```python
from build123d import *

# Parameters (mm, degrees)
BOSS_EXTRUDE1_DEPTH                              = 20.32
BOSS_EXTRUDE2_DEPTH                              = 12.7
CBORE_FOR_10_PAN_HEAD_MACHINE_SCREW1_D           = 5.08
CBORE_FOR_10_PAN_HEAD_MACHINE_SCREW1_CBORE_D     = 12.7
CBORE_FOR_10_PAN_HEAD_MACHINE_SCREW1_CBORE_DEPTH = 3.3782
FILLET1_R                                        = 5.08
FILLET2_R                                        = 2.54
FILLET3_R                                        = 2.54
FILLET4_R                                        = 2.54


with BuildPart() as part:
    # Sketch1 → Boss-Extrude1 (new, symmetric)
    with BuildSketch(Plane(origin=(0, 0, 0), x_dir=(0, 0, -1), z_dir=(1, 0, 0))):
        Polygon((0, 0), (0, 127), (-10.16, 127), (-10.16, 19.05), (-76.2, 19.05), (-76.2, 31.75), (-88.9, 31.75), (-88.9, 0), align=None)
    extrude(amount=BOSS_EXTRUDE1_DEPTH, both=True)

    # Sketch1<9> → Boss-Extrude2 (add, symmetric)
    with BuildSketch(Plane(origin=(0, 0, 0), x_dir=(0, 0, -1), z_dir=(1, 0, 0))):
        Polygon((-54.61, 19.05), (-10.16, 80.01), (-10.16, 67.31), (-45.349583333, 19.05), align=None)
    extrude(amount=BOSS_EXTRUDE2_DEPTH, both=True)

    # CBORE for #10 Pan Head Machine Screw1 (through all)
    with Locations(Plane.XY.offset(10.16)):
        with Locations((0, 91.44), (0, 114.3)):
            CounterBoreHole(CBORE_FOR_10_PAN_HEAD_MACHINE_SCREW1_D / 2, CBORE_FOR_10_PAN_HEAD_MACHINE_SCREW1_CBORE_D / 2, CBORE_FOR_10_PAN_HEAD_MACHINE_SCREW1_CBORE_DEPTH)

    # Fillet1
    fillet1_edges = [part.edges().sort_by_distance(p)[0] for p in [
        (0, 19.05, 10.16),
    ]]
    fillet(fillet1_edges, radius=FILLET1_R)

    # Fillet2
    fillet2_edges = [part.edges().sort_by_distance(p)[0] for p in [
        (0, 19.05, 76.2),
    ]]
    fillet(fillet2_edges, radius=FILLET2_R)

    # Fillet3
    fillet3_edges = [part.edges().sort_by_distance(p)[0] for p in [
        (0, 0, 88.9),
    ]]
    fillet(fillet3_edges, radius=FILLET3_R)

    # Fillet4
    fillet4_edges = [part.edges().sort_by_distance(p)[0] for p in [
        (0, 31.75, 88.9),
    ]]
    fillet(fillet4_edges, radius=FILLET4_R)


solid = part.part
```
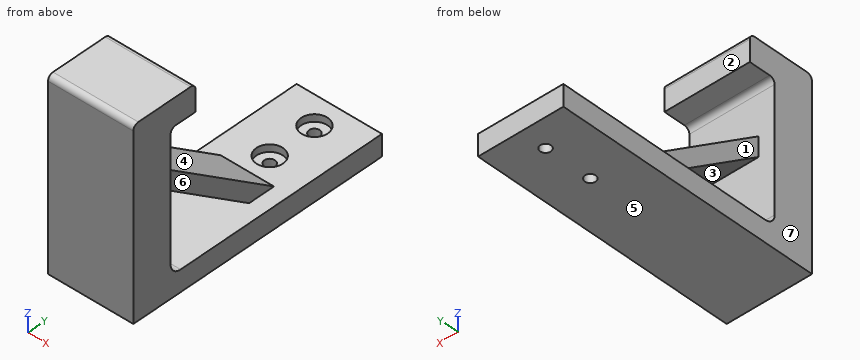
Read the model definition and answer for the solid it produces. Units are mm, in the model's axes. Face numbers are marked on the shaded views. A direction names the side the tool comes from. Coordinates: 2 decimals unless noted, no trailing zeros. Loops run counter-clockwise (first coordinate to the right, second up) from the corner with the lowest first, then second, coordinate; pieces in that order, holes last. Notation, with made-up numbers: (57.25, 51) - (91.25, 51) arc R18 ccw to (91.25, 73) - close; hole circle Ø5 at (5.5, 83.5). An arc over 180 degrees is marked (long way). Answer in a Markdown table with one row per item.
1. Find section C-C, the plane x = -15.5. Write down the section's boundary in (y, z).
Conclusion:
| item | result |
|---|---|
| outline | (0, 0) - (127, 0) - (127, 10.16) - (24.13, 10.16) arc R5.08 cw to (19.05, 15.24) - (19.05, 73.66) arc R2.54 cw to (21.59, 76.2) - (31.75, 76.2) - (31.75, 86.36) arc R2.54 ccw to (29.21, 88.9) - (2.54, 88.9) arc R2.54 ccw to (0, 86.36) - close |
2. Find section D-D, the plane z = 40. Write down the section's boundary in (x, y), then the cut area to 3 significant figures.
Conclusion:
| item | result |
|---|---|
| outline | (-20.32, 0) - (20.32, 0) - (20.32, 19.05) - (-20.32, 19.05) - close; (-12.7, 26.39) - (12.7, 26.39) - (12.7, 39.09) - (-12.7, 39.09) - close |
| area | 1,100 mm² |
3. Given pin 1 (20.5 mm diameter, centred on x = -10, y = 53, fed in from +Z); pin 2 (3 mm diameter, centred on x = -3.5, z = 81, fed in from +Y); pin 3 (14 mm diameter, centred on x = 1.5, y = 116, fed in from +Z); pin 4 (4.5 mm diameter, centred on x = 0, y = 114.3, fed in from -Z), each flat-ended and moving along its own axis, determine where each tip first touches the part or whether it passes through.
Conclusion:
| item | result |
|---|---|
| pin 1 | stops at z = 37.33 |
| pin 2 | stops at y = 31.75 |
| pin 3 | stops at z = 10.16 |
| pin 4 | passes through |
4. Determine the mould class of the marked faces 5, 6 and 7 for opening direction Z: +Z half, -Z half, draft (parallel to the pull), parting line (faces both ways), or undercut.
Conclusion:
| item | result |
|---|---|
| face 5 | -Z half |
| face 6 | undercut |
| face 7 | draft |
5. Find section A-A, the plane y = 91.44. Write down the section's boundary in (x, z), then the cut area to 3 significant figures.
Conclusion:
| item | result |
|---|---|
| outline | (-20.32, 0) - (-2.54, 0) - (-2.54, 6.78) - (-6.35, 6.78) - (-6.35, 10.16) - (-20.32, 10.16) - close; (2.54, 0) - (20.32, 0) - (20.32, 10.16) - (6.35, 10.16) - (6.35, 6.78) - (2.54, 6.78) - close |
| area | 336 mm² |
6. Find section B-B, the plane x = 0. Count the separate pieces of the cut face and the enclosed holes in it, then the cut area to 3 significant figures.
Conclusion:
| item | result |
|---|---|
| separate pieces | 3 |
| enclosed holes | 1 |
| area | 3,310 mm² |
7. Straight lines are drawn through the part: line 1 (Y direction, x = 0, z = 5); line 2 (Y direction, x = 0, z = 8.7); line 3 (X direction, y = 91, z = 9). For each, find the intervals that lie inside material, in ascending order.
Conclusion:
| item | result |
|---|---|
| line 1 | y = 0 to 88.9, 93.98 to 111.76, 116.84 to 127 |
| line 2 | y = 0 to 85.09, 97.79 to 107.95, 120.65 to 127 |
| line 3 | x = -20.32 to -6.33, 6.33 to 20.32 |
8. Which of the six approach directions +Z, -Z, +X, -X, +Y, -Y give full straight-line access (tool end or side, diameter ignored) to the marked faces 1, 2, 3 and 4?
Conclusion:
| item | result |
|---|---|
| face 1 | -X, +Y |
| face 2 | +Z, +X, -X, +Y |
| face 3 | +X, -X |
| face 4 | +X, -X, +Y |
